Work out the finished part from the listing and answer in its coordinate system (mm). Coordinates: 2 decimals unless noted, no trailing zeros. Order: outer loops, then holes, each group sorted by start corner. A loop starts at its lowest first (then second) coordinate and runs counter-clockwise, first axis right, second up.
```python
from build123d import *

# Parameters (mm, degrees)
SKETCH1_W                   = 14
SKETCH1_H                   = 16
BOSS_EXTRUDE1_DEPTH         = 8
TAP_DRILL_FOR_M5X0_8_TAP1_D = 4.2
F_5_0_5_DIAMETER_HOLE1_D    = 5
F_2_1_2_1_DIAMETER_HOLE1_D  = 2.1


with BuildPart() as part:
    # Sketch1 → Boss-Extrude1 (new body)
    with BuildSketch(Plane.XY):
        with Locations((7, 8)):
            Rectangle(SKETCH1_W, SKETCH1_H)
    extrude(amount=BOSS_EXTRUDE1_DEPTH)

    # Tap Drill for M5x0.8 Tap1 (through all)
    with Locations(Plane.XY.offset(8)):
        with Locations((9.5, 12)):
            Hole(TAP_DRILL_FOR_M5X0_8_TAP1_D / 2)

    # Ø5.0 (5) Diameter Hole1 (through all)
    with Locations(Plane.ZY):
        with Locations((4, 4)):
            Hole(F_5_0_5_DIAMETER_HOLE1_D / 2)

    # Ø2.1 (2.1) Diameter Hole1 (through all)
    with Locations(Plane.ZY):
        with Locations((5.85, 7.75)):
            Hole(F_2_1_2_1_DIAMETER_HOLE1_D / 2)


solid = part.part
```
1. The part is cut by section B-B (z = 5.85). Determine the outline of the cut face in (x, y), plus the area to 3 significant figures.
2. The part is cut by section D-D (x = 1.25). Determine the outline of the cut face in (y, z), plus the area to 3 significant figures.
3. The part is cut by section C-C (y = 7.75). Determine the outline of the cut face in (x, z), plus the area to 3 significant figures.
4. A flat-ended cylindrical pin translates along its axis: pin 1 (4 mm diameter, centred on y = 4, z = 4, fed in from -X). Find the tip coordinate at first contact, or state that the pin passes through.
5. Consider probe 1 along Y at (x, z) = (4, 5.85); probe 2 along Y at (x, z) = (5.5, 5); probe 3 along Y at (x, z) = (7, 4). Determine where each line is inside the solid, lowest interval first.
6. The part is cut by section A-A (z = 2). Determine the outline of the cut face in (x, y), plus the area to 3 significant figures.
7. The mould has two halves that part along Y. Classify faces 1 (the flat face through (0, 8, 4)), 2 (the flat face through (7, 16, 4)), 3 (the flat face through (7, 0, 4)), 4 (the cylindrical face through (7.1, 8.64, 5.29)): released by +Y, released by -Y, zero draft, split by the parting line, or undercut.
Worked out:
1. outline: (0, 0) - (14, 0) - (14, 2.32) - (0, 2.32) - close; (0, 5.68) - (14, 5.68) - (14, 6.7) - (0, 6.7) - close; (0, 8.8) - (14, 8.8) - (14, 16) - (0, 16) - close; hole circle Ø4.2 at (9.5, 12)
1. area: 134 mm2
2. outline: (0, 0) - (16, 0) - (16, 8) - (0, 8) - close; hole circle Ø5 at (4, 4); hole circle Ø2.1 at (7.75, 5.85)
2. area: 105 mm2
3. outline: (0, 0) - (14, 0) - (14, 4.8) - (0, 4.8) - close; (0, 6.9) - (14, 6.9) - (14, 8) - (0, 8) - close
3. area: 82.6 mm2
4. pin 1: passes through
5. probe 1: y = 0 to 2.32, 5.68 to 6.7, 8.8 to 16
5. probe 2: y = 0 to 1.71, 6.29 to 7.13, 8.37 to 16
5. probe 3: y = 0 to 1.5, 6.5 to 16
6. outline: (0, 0) - (14, 0) - (14, 2.5) - (0, 2.5) - close; (0, 5.5) - (14, 5.5) - (14, 16) - (0, 16) - close; hole circle Ø4.2 at (9.5, 12)
6. area: 168 mm2
7. face 1: zero draft
7. face 2: released by +Y
7. face 3: released by -Y
7. face 4: undercut
